```python
from build123d import *

# Parameters (mm, degrees)
EXTRUDE_1_DEPTH     = 30
SKETCH_2_W          = 18
SKETCH_2_H          = 28
SKETCH_2_R          = 1.6
EXTRUDE_2_DEPTH     = 3
SKETCH_3_W          = 1.1
SKETCH_3_H          = 6
CUT_EXTRUDE_1_DEPTH = 15
FILLET_1_R          = 3
EXTRUDE_3_DEPTH     = 1.5
SKETCH_6_W          = 8
SKETCH_6_H          = 7.1
EXTRUDE_4_DEPTH     = 30
SKETCH_7_W          = 18
SKETCH_7_H          = 30
CUT_EXTRUDE_3_DEPTH = 10.5
EXTRUDE_5_DEPTH     = 10
CUT_EXTRUDE_5_REACH = 24.392
SKETCH_9_W          = 18
SKETCH_9_H          = 16
CUT_EXTRUDE_6_REACH = 16.731
SKETCH_11_R         = 0.85
SHELL_START         = -20.5
SHELL_1_OUTLINE_W   = 15
SHELL_1_OUTLINE_H   = 10
SHELL_1_OUTLINE_R   = 2.35
SHELL_1_DEPTH       = 4.5
RIB_1_REACH         = 20.028
SKETCH_12_WALLS_W   = 1.5
SKETCH_12_WALLS_H   = 42.055512754


# Read off the part's stored shape, not the designer's step: 抽壳1
with BuildPart() as part:
    # 草图1 → 凸台-拉伸1 (new body)
    with BuildSketch(Plane(origin=(0, 0, 0), x_dir=(1, 0, 0), z_dir=(0, 1, 0))):
        Polygon((-9, 10.1), (-9, 0), (9, 0), (9, 10.1), (4, 10.1), (4, 3), (-4, 3), (-4, 10.1), align=None)
    extrude(amount=EXTRUDE_1_DEPTH)

    # 草图2 → 凸台-拉伸2 (add)
    with BuildSketch(Plane.XZ):
        with Locations((0, -14)):
            Rectangle(SKETCH_2_W, SKETCH_2_H)
        with Locations(Location((4, -25, 0), (0, 0, 270))):
            Circle(SKETCH_2_R, mode=Mode.SUBTRACT)
        with Locations(Location((-4, -25, 0), (0, 0, 270))):
            Circle(SKETCH_2_R, mode=Mode.SUBTRACT)
    extrude(amount=EXTRUDE_2_DEPTH)

    # 草图3 → 切除-拉伸1 (cut)
    with BuildSketch(Plane(origin=(0, 30, 0), x_dir=(1, 0, 0), z_dir=(0, 1, 0))):
        with Locations((-6.95, 7.1)):
            Rectangle(SKETCH_3_W, SKETCH_3_H)
        with Locations((6.95, 7.1)):
            Rectangle(SKETCH_3_W, SKETCH_3_H)
    extrude(amount=-CUT_EXTRUDE_1_DEPTH, mode=Mode.SUBTRACT)

    # 圆角1
    fillet_1_edges = [part.edges().sort_by_distance(p)[0] for p in [
        (9, -1.5, -28),
        (-9, -1.5, -28),
    ]]
    fillet(fillet_1_edges, radius=FILLET_1_R)

    # 草图5 → 凸台-拉伸3 (add)
    with BuildSketch(Plane.ZY.offset(9)):
        Polygon((-10.1, 0), (-10.1, 6), (-15.1, 0), align=None)
    extrude_3 = extrude(amount=-EXTRUDE_3_DEPTH)

    # 镜向1: 凸台-拉伸3 across plane
    add(extrude_3.mirror(Plane(origin=(0, 0, 0), x_dir=(0, 0, 1), z_dir=(1, 0, 0))))

    # 草图6 → 凸台-拉伸4 (add)
    with BuildSketch(Plane(origin=(0, 0, 0), x_dir=(1, 0, 0), z_dir=(0, 1, 0))):
        with Locations((0, 6.55)):
            Rectangle(SKETCH_6_W, SKETCH_6_H)
    extrude(amount=EXTRUDE_4_DEPTH)

    # 草图7 → 切除-拉伸3 (cut, symmetric)
    with BuildSketch(Plane(origin=(0, 0, -10.1), x_dir=(-1, 0, 0), z_dir=(0, 0, -1))):
        with Locations((0, 15)):
            Rectangle(SKETCH_7_W, SKETCH_7_H)
    extrude(amount=CUT_EXTRUDE_3_DEPTH, both=True, mode=Mode.SUBTRACT)

    # 草图10 → 凸台-拉伸5 (add)
    with BuildSketch(Plane(origin=(0, 0, 0), x_dir=(1, 0, 0), z_dir=(0, 1, 0))):
        Polygon((9, 16), (-9, 16), (-9, 24), (-7.5, 24), (-7.5, 22), (7.5, 22), (7.5, 24), (9, 24), align=None)
    extrude(amount=EXTRUDE_5_DEPTH)

    # 草图9 → 切除-拉伸5 (cut, up to next)
    with BuildSketch(Plane(origin=(0, 0, -10.1), x_dir=(-1, 0, 0), z_dir=(0, 1, 0)), mode=Mode.PRIVATE) as cut_extrude_5_sk1:
        with Locations((0, 2.1)):
            Rectangle(SKETCH_9_W, SKETCH_9_H)
    cut_extrude_5_tool1 = extrude(cut_extrude_5_sk1.sketch, amount=-CUT_EXTRUDE_5_REACH, mode=Mode.PRIVATE) & part.part
    add(cut_extrude_5_tool1.solids().sort_by_distance((0, 0, -8))[0], mode=Mode.SUBTRACT)

    # 草图11 → 切除-拉伸6 (cut, up to next)
    with BuildSketch(Plane(origin=(0, 0, -22), x_dir=(-1, 0, 0), z_dir=(0, 0, -1)), mode=Mode.PRIVATE) as cut_extrude_6_sk1:
        with Locations((4, 6)):
            Circle(SKETCH_11_R)
    cut_extrude_6_tool1 = extrude(cut_extrude_6_sk1.sketch, amount=-CUT_EXTRUDE_6_REACH, mode=Mode.PRIVATE) & part.part
    # 草图11 → 切除-拉伸6 (cut, up to next)
    with BuildSketch(Plane(origin=(0, 0, -22), x_dir=(-1, 0, 0), z_dir=(0, 0, -1)), mode=Mode.PRIVATE) as cut_extrude_6_sk2:
        with Locations((-4, 6)):
            Circle(SKETCH_11_R)
    cut_extrude_6_tool2 = extrude(cut_extrude_6_sk2.sketch, amount=-CUT_EXTRUDE_6_REACH, mode=Mode.PRIVATE) & part.part
    add(cut_extrude_6_tool1.solids().sort_by_distance((-4, 6, -22))[0], mode=Mode.SUBTRACT)
    add(cut_extrude_6_tool2.solids().sort_by_distance((4, 6, -22))[0], mode=Mode.SUBTRACT)

    # 抽壳1 outline → 抽壳1 (cut)
    with BuildSketch(Plane.XY.offset(SHELL_START)):
        with Locations((0, 3.5)):
            Rectangle(SHELL_1_OUTLINE_W, SHELL_1_OUTLINE_H)
        with Locations((-4, 6)):
            Circle(SHELL_1_OUTLINE_R, mode=Mode.SUBTRACT)
        with Locations((4, 6)):
            Circle(SHELL_1_OUTLINE_R, mode=Mode.SUBTRACT)
    extrude(amount=SHELL_1_DEPTH, mode=Mode.SUBTRACT)

    # 草图12 walls → 筋1 (add, up to next)
    with BuildSketch(Plane.XY.offset(-16), mode=Mode.PRIVATE) as rib_1_sk1:
        with Locations((4, 8)):
            Rectangle(SKETCH_12_WALLS_W, SKETCH_12_WALLS_H)
    rib_1_tool1 = extrude(rib_1_sk1.sketch, amount=-RIB_1_REACH, mode=Mode.PRIVATE) - part.part
    # 草图12 walls → 筋1 (add, up to next)
    with BuildSketch(Plane.XY.offset(-16), mode=Mode.PRIVATE) as rib_1_sk2:
        with Locations((-4, 8)):
            Rectangle(SKETCH_12_WALLS_W, SKETCH_12_WALLS_H)
    rib_1_tool2 = extrude(rib_1_sk2.sketch, amount=-RIB_1_REACH, mode=Mode.PRIVATE) - part.part
    add(rib_1_tool1.solids().sort_by_distance((4, 8, -16))[0])
    add(rib_1_tool2.solids().sort_by_distance((-4, 8, -16))[0])


solid = part.part
```
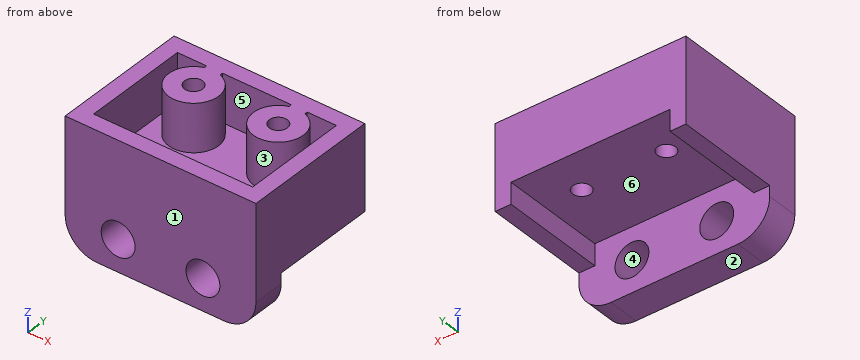
Geometry check sheet. Reference: the model listing, model coordinates, mm. Face numbers are marked on the shaded views. A direction names the side the tool comes from. Round coordinates to 2 decimals unless told otherwise and drop trailing zeros. Loops run counter-clockwise (first coordinate to the right, second up) from the corner with the lowest first, then second, coordinate; pieces in that order, holes last. Notation, with made-up numbers: (71, 58.5) - (115, 58.5) arc R8 ccw to (115, 68.5) - close; hole circle Ø5 at (-40, -1). An arc over 180 degrees is marked (long way). Use a Markdown table: item, result.
Q1. Cross-section at D-D on y = 9.25. Record the cut outline in (x, z), plus the area to 3 significant figures.
Solutions:
| item | result |
|---|---|
| outline | (-9, -24) - (-7.5, -24) - (-7.5, -22) - (7.5, -22) - (7.5, -24) - (9, -24) - (9, -16) - (-9, -16) - close |
| area | 114 mm2 |
Q2. Go/stop test with flat-tipped pins: P1, Ø4, axis at x = 0.5, y = 5.5, coming from the +Z side; P2, Ø2, axis at x = -4, y = 6, coming from the -Z side; P3, Ø3, axis at x = 4, z = -25.5, coming from the +Y side. Record where each tip stops, or that it passes through.
Solutions:
| item | result |
|---|---|
| P1 | stops at z = -16 |
| P2 | stops at z = -22 |
| P3 | stops at y = 0 |
Q3. Material ranges on line 1 (X direction, y = -2.2, z = -25); line 2 (X direction, y = 4.5, z = -23.25); line 3 (X direction, y = 7, z = -20), recorded low to high.
Solutions:
| item | result |
|---|---|
| line 1 | x = -9 to -5.6, -2.4 to 2.4, 5.6 to 9 |
| line 2 | x = -9 to -7.5, 7.5 to 9 |
| line 3 | x = -9 to -7.5, -6.13 to -1.87, 1.87 to 6.13, 7.5 to 9 |
Q4. Cross-section at B-B on y = 6. Record the cut outline in (x, z).
Solutions:
| item | result |
|---|---|
| outline | (-9, -24) - (-7.5, -24) - (-7.5, -22) - (-4.85, -22) - (-4.85, -16) - (-6.35, -16) - (-6.35, -20.5) - (-7.5, -20.5) - (-7.5, -16) - (-9, -16) - close; (-3.15, -22) - (3.15, -22) - (3.15, -16) - (1.65, -16) - (1.65, -20.5) - (-1.65, -20.5) - (-1.65, -16) - (-3.15, -16) - close; (4.85, -22) - (7.5, -22) - (7.5, -24) - (9, -24) - (9, -16) - (7.5, -16) - (7.5, -20.5) - (6.35, -20.5) - (6.35, -16) - (4.85, -16) - close |
Q5. Draft check along Y on the marked faces 1, 2 and 3. Enter one of: released by +Y, released by -Y, zero draft, split by the parting line, or undercut.
Solutions:
| item | result |
|---|---|
| face 1 | released by -Y |
| face 2 | zero draft |
| face 3 | undercut |
Q6. Access from +Z, -Z, +X, -X, +Y, -Y to the whole of each face (thin tool, end or side, straight path). Record for the marked faces 4, 5 and 6.
Solutions:
| item | result |
|---|---|
| face 4 | +Y, -Y |
| face 5 | +Z |
| face 6 | -Z, +Y |
Q7. Cross-section at C-C on z = -19. Record the cut outline in (x, y).
Solutions:
| item | result |
|---|---|
| outline | (-9, -3) - (9, -3) - (9, 10) - (-9, 10) - close; hole (-7.5, -1.5) - (7.5, -1.5) - (7.5, 8.5) - (4.75, 8.5) - (4.75, 8.23) arc R2.35 cw (long way) to (3.25, 8.23) - (3.25, 8.5) - (-3.25, 8.5) - (-3.25, 8.23) arc R2.35 cw (long way) to (-4.75, 8.23) - (-4.75, 8.5) - (-7.5, 8.5) - close; hole circle Ø1.7 at (-4, 6); hole circle Ø1.7 at (4, 6) |
Q8. Cross-section at A-A on x = -4. Record the cut outline in (y, z).
Solutions:
| item | result |
|---|---|
| outline | (-3, -28) - (0, -28) - (0, -26.6) - (-3, -26.6) - close; (-3, -23.4) - (0, -23.4) - (0, -22) - (5.15, -22) - (5.15, -16) - (3.65, -16) - (3.65, -20.5) - (-1.5, -20.5) - (-1.5, -16) - (-3, -16) - close; (6.85, -22) - (10, -22) - (10, -16) - (6.85, -16) - close |
